Can you work these out from the model? Positions are in its coordinate system, mm. Face numbers are marked on the shaded views. A direction names the side the tool comes from. Give positions to 0.01 mm unless a question says otherwise; leave off trailing zeros. Loops run counter-clockwise (first coordinate to the right, second up) from the corner with the lowest first, then second, coordinate; pieces in that order, holes last.
from build123d import *

# Parameters (mm, degrees)
BOSS_EXTRUDE2_DEPTH = 16.8
SKETCH5_R           = 4
CUT_EXTRUDE3_DEPTH  = 38.5
SKETCH6_W           = 20
SKETCH6_H           = 7
CUT_EXTRUDE4_DEPTH  = 2
SKETCH8_W           = 20
SKETCH8_H           = 7
CUT_EXTRUDE5_DEPTH  = 2
CUT_EXTRUDE8_DEPTH  = 3


with BuildPart() as part:
    # Sketch1 → Boss-Extrude2 (new body)
    with BuildSketch(Plane(origin=(0, 0, 0), x_dir=(1, 0, 0), z_dir=(0, 1, 0))):
        Polygon((2.5, -14.25), (-2.5, -14.25), (-57.5, -14.25), (-57.5, -19.25), (2.5, -19.25), align=None)
        Polygon((2.5, 14.25), (-2.5, 14.25), (-2.5, -0.75), (-2.5, -14.25), (2.5, -14.25), align=None)
        Polygon((-57.5, 14.25), (-2.5, 14.25), (2.5, 14.25), (2.5, 19.25), (-57.5, 19.25), align=None)
    extrude(amount=-BOSS_EXTRUDE2_DEPTH)

    # Sketch5 → Cut-Extrude3 (cut)
    with BuildSketch(Plane.XY.offset(19.25)):
        with Locations((-47.5, -8.4)):
            Circle(SKETCH5_R)
    extrude(amount=-CUT_EXTRUDE3_DEPTH, mode=Mode.SUBTRACT)

    # Sketch6 → Cut-Extrude4 (cut)
    with BuildSketch(Plane.XY.offset(19.25)):
        with Locations((-37.5, -8.4)):
            Rectangle(SKETCH6_W, SKETCH6_H)
    extrude(amount=-CUT_EXTRUDE4_DEPTH, mode=Mode.SUBTRACT)

    # Sketch8 → Cut-Extrude5 (cut)
    with BuildSketch(Plane(origin=(0, 0, -19.25), x_dir=(-1, 0, 0), z_dir=(0, 0, -1))):
        with Locations((37.5, -8.492973944)):
            Rectangle(SKETCH8_W, SKETCH8_H)
    extrude(amount=-CUT_EXTRUDE5_DEPTH, mode=Mode.SUBTRACT)

    # Sketch9 → Cut-Extrude8 (cut)
    with BuildSketch(Plane(origin=(2.5, 0, 0), x_dir=(0, 0, -1), z_dir=(1, 0, 0))):
        with BuildLine():
            Line((-19.25, -10.011044161), (-0.79368081, -12.013871992))
            ThreePointArc((-0.79368081, -12.013871992), (-3.696113756, -8.2304621), (-0.459513041, -4.728644969))
            Line((-0.459513041, -4.728644969), (-19.25, -5.9))
            Line((-19.25, -5.9), (-19.25, -10.011044161))
        make_face()
        with BuildLine():
            Line((-0.79368081, -12.013871992), (0, -12.1))
            ThreePointArc((0, -12.1), (2.61629509, -11.01629509), (3.7, -8.4))
            ThreePointArc((3.7, -8.4), (2.61629509, -5.78370491), (0, -4.7))
            Line((0, -4.7), (-0.459513041, -4.728644969))
            ThreePointArc((-0.459513041, -4.728644969), (-3.696113756, -8.2304621), (-0.79368081, -12.013871992))
        make_face()
    extrude(amount=-CUT_EXTRUDE8_DEPTH, mode=Mode.SUBTRACT)


solid = part.part
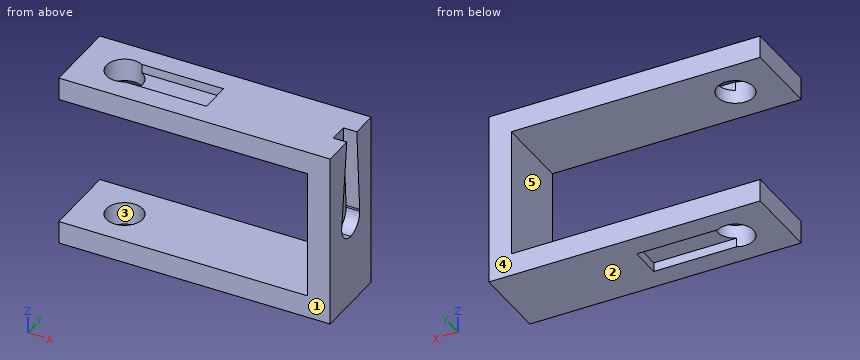
(1) Which directions (+Z, -Z, +X, -X, +Y, -Y) give clear straight access to the entire face, cutting with the end or side of a thin tool? Please do the marked faces 4 and 5.
Returned:
face 4: +Z, -Z, +X, -X, +Y
face 5: -X, +Y, -Y
(2) Suppose I cut it at A-A on x = -11. List the corners of the cut face in (y, z) for me, plus the area to 3 significant figures.
Returned:
outline: (-16.8, -19.25) - (0, -19.25) - (0, -14.25) - (-16.8, -14.25) - close; (-16.8, 14.25) - (0, 14.25) - (0, 19.25) - (-16.8, 19.25) - close
area: 168 mm2
(3) Suppose I cut it at D-D on z = -3. List the corners of the cut face in (x, y) for me.
Returned:
outline: (-2.5, -16.8) - (2.5, -16.8) - (2.5, -10.57) - (-0.5, -10.57) - (-0.5, -6.23) - (2.5, -6.23) - (2.5, 0) - (-2.5, 0) - close
(4) Suppose I cut it at B-B on x = -47.5. List the corners of the cut face in (y, z) for me, plus the area to 3 significant figures.
Returned:
outline: (-16.8, -19.25) - (-12.4, -19.25) - (-12.4, -14.25) - (-16.8, -14.25) - close; (-16.8, 14.25) - (-12.4, 14.25) - (-12.4, 19.25) - (-16.8, 19.25) - close; (-4.4, -19.25) - (0, -19.25) - (0, -14.25) - (-4.4, -14.25) - close; (-4.4, 14.25) - (0, 14.25) - (0, 19.25) - (-4.4, 19.25) - close
area: 88.0 mm2
(5) Please list where these lines run through material, in increasing order: probe 1 along Y at (x, z) = (-47.5, 18.15); probe 2 along X at (y, z) = (-8.4, 18); probe 3 along Z at (x, y) = (-35.5, -5.5).
Returned:
probe 1: y = -16.8 to -12.4, -4.4 to 0
probe 2: x = -57.5 to -51.5, -27.5 to -0.5
probe 3: z = -17.25 to -14.25, 14.25 to 17.25
(6) Will these pins go through, and if not, where does the flat tip stop? P1, Ø1.5, axis at y = -4.5, z = -10, coming from the -X side; P2, Ø2, axis at y = -7, z = 10.5, coming from the +X side; P3, Ø2, axis at x = -33.5, y = -8, coming from the +Z side.
Returned:
P1: stops at x = -2.5
P2: stops at x = -0.5
P3: stops at z = 17.25
(7) Suppose I cut it at C-C on y = -10.75. List the corners of the cut face in (x, z) for me, plus the area to 3 significant figures.
Returned:
outline: (-57.5, -19.25) - (-50.74, -19.25) - (-50.74, -14.25) - (-57.5, -14.25) - close; (-57.5, 14.25) - (-50.74, 14.25) - (-50.74, 19.25) - (-57.5, 19.25) - close; (-44.26, -17.25) - (-27.5, -17.25) - (-27.5, -19.25) - (2.5, -19.25) - (2.5, -2.86) - (-0.5, -2.86) - (-0.5, 12.44) - (2.5, 12.44) - (2.5, 19.25) - (-27.5, 19.25) - (-27.5, 17.25) - (-44.26, 17.25) - (-44.26, 14.25) - (-2.5, 14.25) - (-2.5, -14.25) - (-44.26, -14.25) - close
area: 565 mm2
(8) Thinking about a two-plate mould opening in Y: for the marked faces 1, 2 and 3, which applies, pulls with the +Y half, pulls with the -Y half, needs draft (parallel to the pull), parting line crosses it, or undercut?
Returned:
face 1: pulls with the -Y half
face 2: needs draft
face 3: undercut
